from build123d import *

# Parameters (mm, degrees)
SKETCH1_W               = 24
SKETCH1_H               = 20
BOSS_EXTRUDE1_DEPTH     = 4
SKETCH2_W               = 4
SKETCH2_H               = 20
BOSS_EXTRUDE2_DEPTH     = 20
CHAMFER1_SIZE           = 8
SKETCH3_R               = 1.6
CUT_EXTRUDE1_DEPTH      = 20
SKETCH4_R               = 1.6
CUT_EXTRUDE2_DEPTH      = 20
CHAMFER2_SIZE           = 4
CUT_EXTRUDE3_DEPTH      = 40.395431207
CUT_EXTRUDE3_DEPTH_BACK = 40.395431207
SKETCH5_R               = 2.4


with BuildPart() as part:
    # Sketch1 → Boss-Extrude1 (new body)
    with BuildSketch(Plane(origin=(0, 0, 0), x_dir=(1, 0, 0), z_dir=(0, 1, 0))):
        with Locations((12, 10)):
            Rectangle(SKETCH1_W, SKETCH1_H)
    extrude(amount=BOSS_EXTRUDE1_DEPTH)

    # Sketch2 → Boss-Extrude2 (add)
    with BuildSketch(Plane(origin=(0, 4, 0), x_dir=(1, 0, 0), z_dir=(0, 1, 0))):
        with Locations((2, 10)):
            Rectangle(SKETCH2_W, SKETCH2_H)
    extrude(amount=BOSS_EXTRUDE2_DEPTH)

    # Chamfer1
    chamfer1_edges = [part.edges().sort_by_distance(p)[0] for p in [
        (4, 4, -10),
    ]]
    chamfer(chamfer1_edges, length=CHAMFER1_SIZE)

    # Sketch3 → Cut-Extrude1 (cut)
    with BuildSketch(Plane(origin=(0, 4, 0), x_dir=(1, 0, 0), z_dir=(0, 1, 0))):
        with Locations(Location((18, 10, 0), (0, 0, 270))):
            Circle(SKETCH3_R)
    extrude(amount=-CUT_EXTRUDE1_DEPTH, mode=Mode.SUBTRACT)

    # Sketch4 → Cut-Extrude2 (cut)
    with BuildSketch(Plane(origin=(4, 0, 0), x_dir=(0, 0, -1), z_dir=(1, 0, 0))):
        with Locations((10, 18)):
            Circle(SKETCH4_R)
    extrude(amount=-CUT_EXTRUDE2_DEPTH, mode=Mode.SUBTRACT)

    # Chamfer2
    chamfer2_edges = [part.edges().sort_by_distance(p)[0] for p in [
        (2, 24, 0),
        (2, 24, -20),
        (24, 2, -20),
        (24, 2, 0),
    ]]
    chamfer(chamfer2_edges, length=CHAMFER2_SIZE)

    # Sketch5 → Cut-Extrude3 (cut, two sides: drawn at the far end of the back side and taken through both)
    with BuildSketch(Plane.XY.offset(-CUT_EXTRUDE3_DEPTH_BACK)):
        with Locations((4.818019485, 4.818019485)):
            Circle(SKETCH5_R)
    extrude(amount=CUT_EXTRUDE3_DEPTH + CUT_EXTRUDE3_DEPTH_BACK, mode=Mode.SUBTRACT)


solid = part.part
Geometry: final body of the model. Coordinates: model frame, mm. A direction names the side the tool comes from. Give positions to 0.01 mm unless a question says otherwise; leave off trailing zeros. Loops run counter-clockwise (first coordinate to the right, second up) from the corner with the lowest first, then second, coordinate; pieces in that order, holes last. Notation, with made-up numbers: M 84.25,74 L 138.25,74 A22 ccw 138.25,82 Z; hole C 36,28 d3. An arc over 180 degrees is marked long. Put each result on its own line as item: value.
1) Cut plane D-D, the plane x = 19.25. Return the cut outline in (y, z), plus the area to 3 significant figures.
Computed values:
outline: M 0,-20 L 4,-20 L 4,-11 L 0,-11 Z; M 0,-9 L 4,-9 L 4,0 L 0,0 Z
area: 72.0 mm^2
2) Cut plane C-C, the plane y = 18. Return the cut outline in (x, z).
Computed values:
outline: M 0,-20 L 4,-20 L 4,-11.6 L 0,-11.6 Z; M 0,-8.4 L 4,-8.4 L 4,0 L 0,0 Z
3) Cut plane A-A, the plane z = -10. Return the cut outline in (x, y).
Computed values:
outline: M 0,0 L 16.4,0 L 16.4,4 L 12,4 L 4,12 L 4,16.4 L 0,16.4 Z; M 0,19.6 L 4,19.6 L 4,24 L 0,24 Z; M 19.6,0 L 24,0 L 24,4 L 19.6,4 Z; hole C 4.82,4.82 d4.8
4) First-contact query: P1, Ø1.5, axis at x = 17, z = -15.5, coming from the +Y side; P2, Ø1.5, axis at x = 5.5, y = 18, coming from the -Z side; P3, Ø4, axis at y = 18, z = -10, coming from the +X side. Flat tips, straight axial feed; report the tip coordinate or a pass-through.
Computed values:
P1: stops at y = 4
P2: passes through
P3: stops at x = 4
5) Cut plane B-B, the plane x = 3.25. Return the cut outline in (y, z).
Computed values:
outline: M 0,-20 L 3,-20 L 3,0 L 0,0 Z; M 6.63,-20 L 20,-20 L 24,-16 L 24,-4 L 20,0 L 6.63,0 Z; hole C 18,-10 d3.2
6) Material intervals for L1, parallel to X at y = 2.65, z = -10; L2, parallel to Y at x = 3.75, z = -11; L3, parallel to X at y = 3, z = -10, sorted ascending. Write a range as from..to.
Computed values:
L1: x = 0..3.79, 5.85..16.4, 19.6..24
L2: y = 0..2.67, 6.97..16.75, 19.25..24
L3: x = 0..3.25, 6.38..16.4, 19.6..24
7) Reachability of faces 1 (the flat face through (18, 4, -8)), 2 (the flat face through (2, 24, -10)) from +Z, -Z, +X, -X, +Y, -Y: full face, straight path, thin tool, end or side. Return the list, or none.
Computed values:
face 1: +Z, -Z, +X, +Y
face 2: +Z, -Z, +X, -X, +Y
8) Mould query, pull axis X, two halves, no side actions, for faces 3 (the cylindrical face through (19.586, 2.028, -10.208)), 4 (the flat face through (7.6, 7.6, 0)), 5 (the flat face through (8, 8, -10)), 6 (the flat face through (0, 12, -10)). Classes: released by +X, released by -X, zero draft, split by the parting line, or undercut.
Computed values:
face 3: undercut
face 4: zero draft
face 5: released by +X
face 6: released by -X
